Read the model definition and answer for the solid it produces. Units are mm, in the model's axes. A direction names the side the tool comes from. Give positions to 0.01 mm unless a question says otherwise; leave off trailing zeros. Loops run counter-clockwise (first coordinate to the right, second up) from the corner with the lowest first, then second, coordinate; pieces in that order, holes last. Notation, with made-up numbers: (5.25, 88.25) -> (16.25, 88.25) arc R18 ccw to (16.25, 119.25) -> close; hole circle Ø5 at (85, 8). An arc over 180 degrees is marked (long way). Write each question's results on one line, items separated by ' | '. Start each with the question number.
Item 1: Which of the six approach directions +Z, -Z, +X, -X, +Y, -Y give full straight-line access (tool end or side, diameter ignored) to faces 5 (the flat face through (-12, 16, 15.524)), 6 (the flat face through (-13, 18, 4.739)), 7 (the cylindrical face through (-41.35, 2.52, -0.33))?
Item 2: Find the intervals of material crossed by line 1 (Z direction, x = 5.5, y = -3); line 2 (Y direction, x = 22.5, z = 8.5); line 3 (X direction, y = -1.5, z = 15), in increasing order.
Item 3: Section A-A on x = -31.5 is taken. Write down the section's boundary in (y, z).
Item 4: Each of these flat-tipped pins is pushed along its axis until it touches: P1, Ø1.6, axis at x = -11, y = 16, coming from the +Z side; P2, Ø2.5, axis at x = 12, y = -15.5, coming from the +Z side; P3, Ø4, axis at x = -15, y = 19, coming from the -Z side; P4, Ø10, axis at x = -31.5, y = 15, coming from the -Z side. Where does it stop, or does it pass through?
Item 5: Determine the mould class of faces 1 (the flat face through (27.841, 3, 0)), 2 (the flat face through (1, 0, 26.858)), 3 (the flat face through (0.129, 26.321, 4.346)), 4 (the cylindrical face through (26.459, 1.148, -3.644)) for opening direction X: +X half, -X half, draft (parallel to the pull), parting line (faces both ways), or undercut.
```python
from build123d import *
from build123d.topology import SkipClean

# Parameters (mm, degrees)
SKETCH1_R                = 27.950000405
BOSS_EXTRUDE1_DEPTH      = 27.620221436
FILLET1_R                = 26.67
SHELL1_T                 = -1.778
SKETCH3_W                = 2.977781537
SKETCH3_H                = 2.754447922
BOSS_EXTRUDE3_DEPTH      = 1.016
SKETCH4_R                = 3.820330599
BOSS_EXTRUDE4_DEPTH      = 10.288651178
BOSS_EXTRUDE4_DEPTH_BACK = 82.910790355
SKETCH5_R                = 0.218500346
CUT_EXTRUDE1_DEPTH       = 74.422
SKETCH6_R                = 4.452679147
SKETCH6_R_2              = 2.541856533
CUT_EXTRUDE2_DEPTH       = 26.465589921
SKETCH7_R                = 4.579796813
SKETCH7_R_2              = 2.595326306
CUT_EXTRUDE3_DEPTH       = 10.959776966
SKETCH9_R                = 25.327508304
CUT_EXTRUDE4_DEPTH       = 8.128
CUT_EXTRUDE4_DEPTH_BACK  = 4.572
SKETCH10_R               = 0.226571895
CUT_EXTRUDE5_DEPTH       = 5.588
SKETCH11_R               = 0.957654217
BOSS_EXTRUDE5_DEPTH      = 22.86
SKETCH12_R               = 3.048
BOSS_EXTRUDE6_DEPTH      = 10.78430752
BOSS_EXTRUDE6_2_DEPTH    = 10.78430752
SKETCH14_R               = 2.111885876
CUT_EXTRUDE6_DEPTH       = 33.274
CUT_EXTRUDE7_DEPTH       = 66.802
CUT_EXTRUDE8_DEPTH       = 66.802
SKETCH17_R               = 6.985
CUT_EXTRUDE9_DEPTH       = 0.762
BOSS_EXTRUDE7_DEPTH      = 3.302
BOSS_EXTRUDE8_DEPTH      = 4.572


with BuildPart() as part:
    # Sketch1 → Boss-Extrude1 (new body)
    with BuildSketch(Plane.XY):
        Circle(SKETCH1_R)
    extrude(amount=BOSS_EXTRUDE1_DEPTH)

    # Fillet1
    fillet1_edges = [part.edges().sort_by_distance(p)[0] for p in [
        (-27.950000405, 0, 27.620221436),
    ]]
    fillet(fillet1_edges, radius=FILLET1_R)

    # Shell1
    shell1_openings = [part.faces().sort_by_distance(p)[0] for p in [
        (0, 0, 0),
    ]]
    offset(amount=SHELL1_T, openings=shell1_openings, kind=Kind.INTERSECTION)

    # Sketch3 → Boss-Extrude3 (add)
    with BuildSketch(Plane(origin=(0, 0, 0), x_dir=(-1, 0, 0), z_dir=(0, 0, -1))):
        with Locations((-27.023367447, 0)):
            Rectangle(SKETCH3_W, SKETCH3_H)
    extrude(amount=BOSS_EXTRUDE3_DEPTH)

    # Sketch4 → Boss-Extrude4 (add, two sides)
    with BuildSketch(Plane(origin=(28.512258215, 0, 0), x_dir=(0, 0, -1), z_dir=(1, 0, 0))) as boss_extrude4_sk:
        Circle(SKETCH4_R)
    extrude(amount=BOSS_EXTRUDE4_DEPTH)
    extrude(boss_extrude4_sk.sketch, amount=-BOSS_EXTRUDE4_DEPTH_BACK)

    # Sketch5 → Cut-Extrude1 (cut)
    with BuildSketch(Plane.ZY.offset(54.39853214)):
        Circle(SKETCH5_R)
    extrude(amount=-CUT_EXTRUDE1_DEPTH, mode=Mode.SUBTRACT)

    # Sketch6 → Cut-Extrude2 (cut)
    with BuildSketch(Plane.ZY.offset(54.39853214)):
        Circle(SKETCH6_R)
        Circle(SKETCH6_R_2, mode=Mode.SUBTRACT)
    extrude(amount=-CUT_EXTRUDE2_DEPTH, mode=Mode.SUBTRACT)

    # Sketch7 → Cut-Extrude3 (cut)
    with BuildSketch(Plane(origin=(38.800909393, 0, 0), x_dir=(0, 0, -1), z_dir=(1, 0, 0))):
        Circle(SKETCH7_R)
        Circle(SKETCH7_R_2, mode=Mode.SUBTRACT)
    extrude(amount=-CUT_EXTRUDE3_DEPTH, mode=Mode.SUBTRACT)

    # Sketch9 → Cut-Extrude4 (cut, two sides)
    with BuildSketch(Plane(origin=(0, 0, 0), x_dir=(-1, 0, 0), z_dir=(0, 0, -1))) as cut_extrude4_sk:
        Circle(SKETCH9_R)
    extrude(amount=CUT_EXTRUDE4_DEPTH, mode=Mode.SUBTRACT)
    extrude(cut_extrude4_sk.sketch, amount=-CUT_EXTRUDE4_DEPTH_BACK, mode=Mode.SUBTRACT)

    # Sketch10 → Cut-Extrude5 (cut)
    with BuildSketch(Plane.XY.offset(27.620221436)):
        Circle(SKETCH10_R)
    extrude(amount=-CUT_EXTRUDE5_DEPTH, mode=Mode.SUBTRACT)

    # Sketch15 → Cut-Extrude7 (cut)
    with BuildSketch(Plane(origin=(38.800909393, 0, 0), x_dir=(0, 0, -1), z_dir=(1, 0, 0))):
        Polygon((0, 3.820330599), (-4.891274508, 29.145036791), (1.659844873, 29.145036791), align=None)
    extrude(amount=-CUT_EXTRUDE7_DEPTH, mode=Mode.SUBTRACT)

    # Sketch16 → Cut-Extrude8 (cut)
    with BuildSketch(Plane(origin=(38.800909393, 0, 0), x_dir=(0, 0, -1), z_dir=(1, 0, 0))):
        Polygon((0, -3.820330599), (-4.28892383, -28.486260213), (3.820330599, -28.486260213), align=None)
    extrude(amount=-CUT_EXTRUDE8_DEPTH, mode=Mode.SUBTRACT)

    # Sketch17 → Cut-Extrude9 (cut)
    with BuildSketch(Plane.XY.offset(27.620221436)):
        Circle(SKETCH17_R)
    extrude(amount=-CUT_EXTRUDE9_DEPTH, mode=Mode.SUBTRACT)



with BuildPart() as body_2:
    # Sketch11 → Boss-Extrude5 (new body)
    with BuildSketch(Plane.XY.offset(27.599408823)):
        Circle(SKETCH11_R)
    extrude(amount=-BOSS_EXTRUDE5_DEPTH)

    # Sketch14 → Cut-Extrude6 (cut)
    with BuildSketch(Plane(origin=(0, 0, 0), x_dir=(-1, 0, 0), z_dir=(0, 0, -1))):
        Circle(SKETCH14_R)
    extrude(amount=-CUT_EXTRUDE6_DEPTH, mode=Mode.SUBTRACT)


with BuildPart() as body_3:
    # Sketch12 → Boss-Extrude6 (new body)
    with BuildSketch(Plane(origin=(0, 0, 4.739408823), x_dir=(-1, 0, 0), z_dir=(0, 0, -1))):
        with Locations((11.938, 16.638354337)):
            Circle(SKETCH12_R)
    extrude(amount=-BOSS_EXTRUDE6_DEPTH)


with BuildPart() as body_4:
    # Sketch12 → Boss-Extrude6 2 (new body)
    with BuildSketch(Plane(origin=(0, 0, 4.739408823), x_dir=(-1, 0, 0), z_dir=(0, 0, -1))):
        with Locations((-11.953495285, -16.638354337)):
            Circle(SKETCH12_R)
    extrude(amount=-BOSS_EXTRUDE6_2_DEPTH)


with BuildPart() as part_1:
    add(part.part)

    add(body_3.part)  # Boss-Extrude7 merges body 3
    # Sketch18 → Boss-Extrude7 (add)
    with BuildSketch(Plane(origin=(0, 0, 4.739408823), x_dir=(-1, 0, 0), z_dir=(0, 0, -1))):
        Polygon((9.396577434, 18.321053164), (12.856272932, 23.546318713), (17.452915624, 20.502840084), (14.479422566, 14.95565551), align=None)
    extrude(amount=-BOSS_EXTRUDE7_DEPTH)


    with SkipClean():  # the faces are left unmerged after this step: merging them gives an invalid solid
        add(body_4.part)  # Boss-Extrude8 merges body 4
        # Sketch19 → Boss-Extrude8 (add)
        with BuildSketch(Plane(origin=(0, 0, 4.739408823), x_dir=(-1, 0, 0), z_dir=(0, 0, -1))):
            Polygon((-14.498283748, -14.960750189), (-17.613549805, -19.686354337), (-12.938248054, -22.625591837), (-9.601439985, -18.576946575), align=None)
        extrude(amount=-BOSS_EXTRUDE8_DEPTH)


solid = part_1.part
```
Findings:
1) face 5: none | face 6: -Z | face 7: -X
2) line 1: 25.34 to 26.86 | line 2: -14.67 to -10.9, 10.9 to 14.67 | line 3: -23.9 to -21.78, 21.78 to 23.9
3) outline: circle Ø5.08 at (0, 0); hole circle Ø0.44 at (0, 0)
4) P1: z = 21.22 | P2: z = 21.44 | P3: z = 3.13 | P4: through
5) face 1: +X half | face 2: undercut | face 3: draft | face 4: undercut
